The model under review builds one solid part; all positions refer to its coordinate system, in mm. Face numbers are marked on the shaded views. Round coordinates to 2 decimals unless told otherwise and drop trailing zeros. Write each loop counter-clockwise with the first axis right and the second up, starting at its lowest first coordinate (ties: lowest second). Pieces come first, ordered by that corner, then holes. Notation, with made-up numbers: M -37.5,53.5 L -6.5,53.5 A32 cw -6.5,79.5 Z; hole C 18,-30 d5. An arc over 180 degrees is marked long. Write item = value, one per line. Start each with the question number.
Item 1: For pin 1 Ø1.9 at (x, z) = (0, -12.5) entering from +Y; pin 2 Ø4 at (x, z) = (2, -2.5) entering from +Y; pin 3 Ø8 at (y, z) = (4.5, -6) entering from +X; pin 4 Ø1.5 at (x, z) = (3.5, -12) entering from -Y, all flat-tipped, find the tip position at first contact; note any pin that passes through.
Item 2: The part is to be moulded in two halves that separate along Z. For the marked faces 1, 2 and 3, say which applies: +Z half, -Z half, draft (parallel to the pull), parting line (faces both ways), or undercut.
Item 3: Take a section at B-B, the plane z = 12.5. Give the boundary of the cut face in (x, y) (3 decimals), plus the area to 3 significant figures.
Item 4: Take a section at C-C, the plane z = -8.5. Give the boundary of the cut face in (x, y) (3 decimals).
Item 5: Take a section at A-A, the plane x = 0. Give the boundary of the cut face in (y, z) (3 decimals).
Item 6: Take a section at D-D, the plane y = 2.75. Give the number of separate pieces and of enclosed holes in the cut face, plus the area to 3 significant figures.
Item 7: To check wall thickness, follow line 1 along X through (y, z) = (-3.5, -3); line 2 along X through (y, z) = (1.25, -12.5); line 3 along Z through (x, y) = (3.5, -2.25). State the ranges of each line that lie inside material, in increasing order.
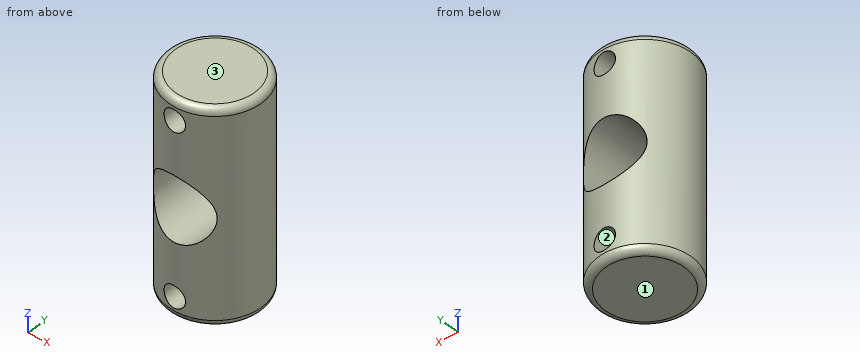
from build123d import *

# Parameters (mm, degrees)
BOSS_EXTRUDE1_DEPTH      = 15.5
BOSS_EXTRUDE1_DEPTH_BACK = 15.5
SKETCH1_R                = 6.825
CUT_EXTRUDE1_DEPTH       = 10
CUT_EXTRUDE1_DEPTH_BACK  = 10
SKETCH2_R                = 4.75
SKETCH2_R_2              = 1.6
FILLET1_R                = 1


with BuildPart() as part:
    # Sketch1 → Boss-Extrude1 (new, two sides: drawn at the far end of the back side and taken through both)
    with BuildSketch(Plane.XY.offset(-BOSS_EXTRUDE1_DEPTH_BACK)):
        Circle(SKETCH1_R)
    extrude(amount=BOSS_EXTRUDE1_DEPTH + BOSS_EXTRUDE1_DEPTH_BACK)

    # Sketch2 → Cut-Extrude1 (cut, two sides: drawn at the far end of the back side and taken through both)
    with BuildSketch(Plane(origin=(0, 0, 0), x_dir=(1, 0, 0), z_dir=(0, 1, 0)).offset(-CUT_EXTRUDE1_DEPTH_BACK)):
        with Locations(Location((0, 0, 0), (0, 0, 90))):
            Circle(SKETCH2_R)
        with Locations(Location((0, -12.5, 0), (0, 0, 90))):
            Circle(SKETCH2_R_2)
        with Locations(Location((0, 12.5, 0), (0, 0, 90))):
            Circle(SKETCH2_R_2)
    extrude(amount=CUT_EXTRUDE1_DEPTH + CUT_EXTRUDE1_DEPTH_BACK, mode=Mode.SUBTRACT)

    # Fillet1
    fillet1_edges = [part.edges().sort_by_distance(p)[0] for p in [
        (-6.825, 0, 15.5),
        (-6.825, 0, -15.5),
    ]]
    fillet(fillet1_edges, radius=FILLET1_R)


solid = part.part
Response values:
q1.pin_1 = through
q1.pin_2 = 6.63
q1.pin_3 = 6.81
q1.pin_4 = -6.25
q2.face_1 = -Z half
q2.face_2 = undercut
q2.face_3 = +Z half
q3.outline = M -1.6,-6.635 L -1.6,6.635 A6.825 ccw Z; M 1.6,-6.635 A6.825 ccw 1.6,6.635 Z
q3.area = 103 mm2
q4.outline = C 0,0 d13.65
q5.outline = M -6.825,-14.5 A1 ccw -5.825,-15.5 L 5.825,-15.5 A1 ccw 6.825,-14.5 L 6.825,-14.1 L -6.825,-14.1 Z; M -6.825,-10.9 L 6.825,-10.9 L 6.825,-4.75 L -6.825,-4.75 Z; M -6.825,4.75 L 6.825,4.75 L 6.825,10.9 L -6.825,10.9 Z; M -6.825,14.1 L 6.825,14.1 L 6.825,14.5 A1 ccw 5.825,15.5 L -5.825,15.5 A1 ccw -6.825,14.5 Z
q6.separate_pieces = 1
q6.enclosed_holes = 3
q6.area = 299 mm2
q7.line_1 = -5.86 to -3.68, 3.68 to 5.86
q7.line_2 = -6.71 to -1.6, 1.6 to 6.71
q7.line_3 = -15.5 to -3.21, 3.21 to 15.5
